Verification items for this drawing (mm, ordinates from the low corner). A direction names the side the tool comes from. Coordinates: 2 decimals unless noted, no trailing zeros. Order: outer loops, then holes, each group sorted by start corner. A loop starts at its lowest first (then second) coordinate and runs counter-clockwise, first axis right, second up. Notation, with made-up numbers: M -38.5,86 L -1.5,86 A16 ccw -1.5,95 Z; hole C 12,62 d1. An arc over 180 degrees is marked long. Answer as a JSON object with one key per item and string values. Group by question number.
(1) Cross-section at A-A (z = 8.5). Enter the section's corners in (x, y).
(2) Material ranges on line 1 (Z direction, x = 27, y = 3.25); line 2 (Z direction, x = 16.5, y = 1), recorded low to high.
(3) Access from +Z, -Z, +X, -X, +Y, -Y to the whole of each face (thin tool, end or side, straight path). Record for the marked faces 1 and 2.
(4) Cross-section at C-C (x = 27). Enter the section's corners in (y, z).
(5) Cross-section at B-B (y = 12). Enter the section's corners in (x, z).
(6) Gauge pin test, flat ends, axial feed: pin 1 Ø1 at (y, z) = (8.5, 53) entering from +X; pin 2 Ø1 at (x, y) = (53, 5.5) entering from +Z; pin 3 Ø0.6 at (y, z) = (8.5, 1) entering from -X. Record the tip position at first contact, or that the pin passes through.
(7) Mould release check, pull along Z, two halves, no side actions. Record for the marked faces 3, 4 and 5: released by +Z, released by -Z, zero draft, split by the parting line, or undercut.
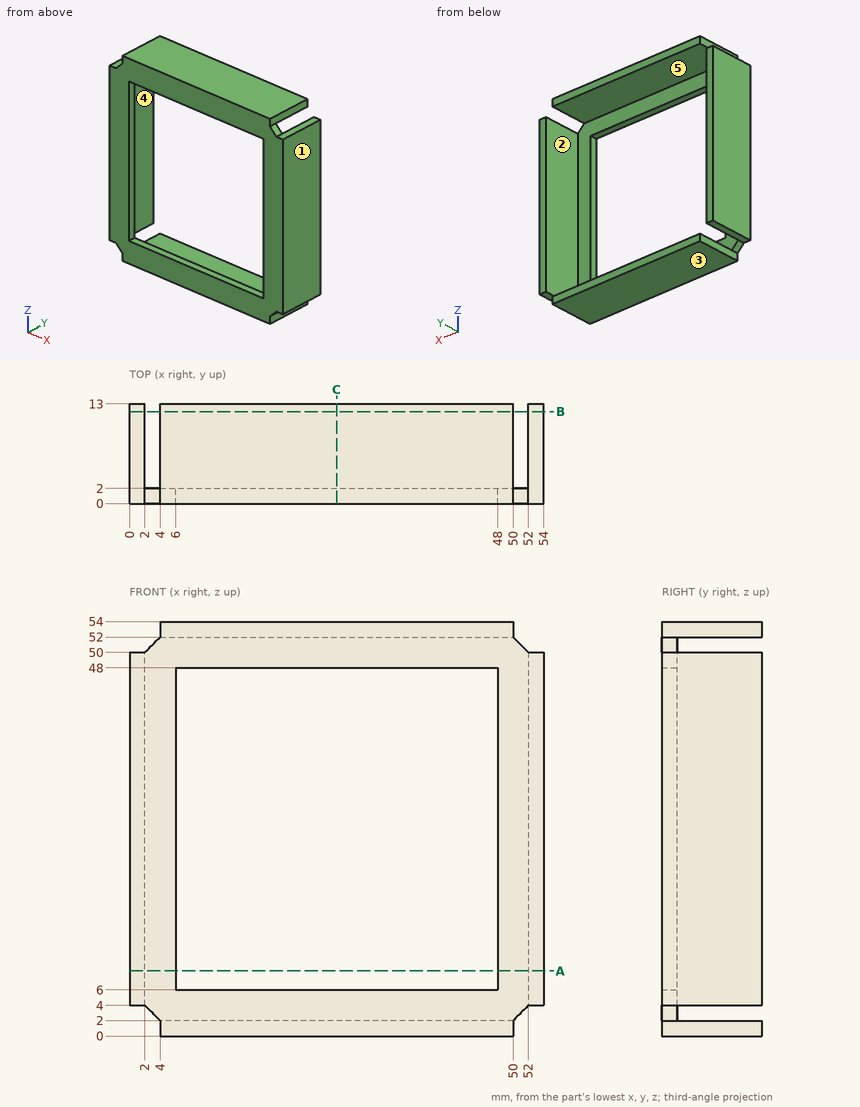
Taken from the geometry:
{
 "1": {"outline": "M 0,0 L 6,0 L 6,2 L 2,2 L 2,13 L 0,13 Z; M 48,0 L 54,0 L 54,13 L 52,13 L 52,2 L 48,2 Z"},
 "2": {"line 1": "z = 0 to 2, 52 to 54", "line 2": "z = 0 to 6, 48 to 54"},
 "3": {"face 1": "+Z, -Z, +X, +Y, -Y", "face 2": "+Z, -Z, +Y"},
 "4": {"outline": "M 0,0 L 13,0 L 13,2 L 2,2 L 2,6 L 0,6 Z; M 0,48 L 2,48 L 2,52 L 13,52 L 13,54 L 0,54 Z"},
 "5": {"outline": "M 0,4 L 2,4 L 2,50 L 0,50 Z; M 4,0 L 50,0 L 50,2 L 4,2 Z; M 4,52 L 50,52 L 50,54 L 4,54 Z; M 52,4 L 54,4 L 54,50 L 52,50 Z"},
 "6": {"pin 1": "stops at x = 50", "pin 2": "stops at z = 50", "pin 3": "stops at x = 4"},
 "7": {"face 3": "released by -Z", "face 4": "zero draft", "face 5": "undercut"}
}
